Could you check a few things on this model? Use its own coordinates, in mm. A direction names the side the tool comes from. Round coordinates to 2 decimals unless told otherwise and drop trailing zeros. Loops run counter-clockwise (first coordinate to the right, second up) from the corner with the lowest first, then second, coordinate; pieces in that order, holes last. Notation, with made-up numbers: (57, 70.5) - (61, 70.5) arc R29 ccw to (61, 101.5) - close; hole circle Ø11 at (49, 80.25). An arc over 180 degrees is marked (long way). Answer as CSV lines item,"result". Start each with the question number.
1) Please list where these lines run through material, in increasing order: line 1 along X through (y, z) = (-6, 9.5); line 2 along X through (y, z) = (-16.5, 3.75); line 3 along Y through (x, z) = (7, 12.5).
2) Suppose I cut it at B-B, the plane z = 2. Write out the boundary of the cut face in (x, y).
3) Suppose I cut it at C-C, the plane x = 5. Write out the boundary of the cut face in (y, z), then the cut area to 3 significant figures.
4) We'd pull the mould along X, two halves only. Please class faces 6 (the face through (12, -16, 7)), 7 (the face through (-2, -4, 15)), 8 (the face through (-2.37, -11.7, 7.41)), 9 (the face through (-8, 0, 7)): pulls with the +X half, pulls with the -X half, needs draft (parallel to the pull), parting line crosses it, or undercut.
5) Suppose I cut it at A-A, the plane y = -4. Write out the boundary of the cut face in (x, z), then the cut area to 3 significant figures.
6) I'm going to push flat-ended pins straight in: pin 1 Ø1 at (y, z) = (9, 12.5) entering from +X; pin 2 Ø8 at (y, z) = (-17, 7) entering from -X; pin 3 Ø4 at (x, z) = (-2, 5.5) entering from -Y. Where does each tip first touch, or does it pass through?
7) Which directions (+Z, -Z, +X, -X, +Y, -Y) give clear straight access to the entire face, cutting with the end or side of a thin tool? Please do faces 1 (the face through (-4.5, -2.8, 0.5)), 2 (the face through (8.5, -16.2, 14.5)), 3 (the face through (-3.5, -10.84, 0.49)), 4 (the face through (2, -6, 7)), 5 (the face through (-1.5, -15.9, 14.5)).
```python
from build123d import *

# Parameters (mm, degrees)
F1_DEPTH = 15
F2_SIZE  = 1


with BuildPart() as f1:
    # F0 (on Top) → F1 (new body)
    with BuildSketch(Plane.XY):
        with BuildLine():
            ThreePointArc((-8, 8.423196), (-8.585786, 7.008983), (-10, 6.423196))
            Line((-10, 6.423196), (-10, -7.990119))
            Line((-10, -7.990119), (-10, -9.990119))
            ThreePointArc((-10, -9.990119), (-8.585786, -9.404332), (-8, -7.990119))
            Line((-8, -7.990119), (-8, 8.423196))
        make_face()
        with BuildLine():
            Line((-10, -7.990119), (-10, 6.423196))
            ThreePointArc((-10, 6.423196), (-11.414214, 7.008983), (-12, 8.423196))
            Line((-12, 8.423196), (-12, -7.990119))
            ThreePointArc((-12, -7.990119), (-11.414214, -9.404332), (-10, -9.990119))
            Line((-10, -9.990119), (-10, -7.990119))
        make_face()
        with BuildLine():
            Line((-10, 6.423196), (-10, 8.423196))
            ThreePointArc((-10, 8.423196), (-9.898979, 9.423196), (-9.6, 10.382788))
            ThreePointArc((-9.6, 10.382788), (-11.264911, 9.97239), (-12, 8.423196))
            ThreePointArc((-12, 8.423196), (-11.414214, 7.008983), (-10, 6.423196))
        make_face()
        with BuildLine():
            ThreePointArc((-9.6, 10.382788), (-9.898979, 9.423196), (-10, 8.423196))
            Line((-10, 8.423196), (-10, 6.423196))
            ThreePointArc((-10, 6.423196), (-8.585786, 7.008983), (-8, 8.423196))
            ThreePointArc((-8, 8.423196), (-8.450807, 9.688108), (-9.6, 10.382788))
        make_face()
        with BuildLine():
            ThreePointArc((-0.4, 10.382788), (-5, 13.423196), (-9.6, 10.382788))
            ThreePointArc((-9.6, 10.382788), (-8.450807, 9.688108), (-8, 8.423196))
            ThreePointArc((-8, 8.423196), (-5, 11.423196), (-2, 8.423196))
            ThreePointArc((-2, 8.423196), (-1.549193, 9.688108), (-0.4, 10.382788))
        make_face()
        with BuildLine():
            ThreePointArc((-12, 8.423196), (-11.264911, 9.97239), (-9.6, 10.382788))
            ThreePointArc((-9.6, 10.382788), (-5, 13.423196), (-0.4, 10.382788))
            ThreePointArc((-0.4, 10.382788), (1.264911, 9.97239), (2, 8.423196))
            ThreePointArc((2, 8.423196), (-5, 15.423196), (-12, 8.423196))
        make_face()
        with BuildLine():
            ThreePointArc((2, 8.423196), (1.264911, 9.97239), (-0.4, 10.382788))
            ThreePointArc((-0.4, 10.382788), (-0.101021, 9.423196), (0, 8.423196))
            Line((0, 8.423196), (0, 6.423196))
            ThreePointArc((0, 6.423196), (1.414214, 7.008983), (2, 8.423196))
        make_face()
        with BuildLine():
            ThreePointArc((0, 8.423196), (-0.101021, 9.423196), (-0.4, 10.382788))
            ThreePointArc((-0.4, 10.382788), (-1.549193, 9.688108), (-2, 8.423196))
            ThreePointArc((-2, 8.423196), (-1.414214, 7.008983), (0, 6.423196))
            Line((0, 6.423196), (0, 8.423196))
        make_face()
        with BuildLine():
            ThreePointArc((0, 6.423196), (-1.414214, 7.008983), (-2, 8.423196))
            ThreePointArc((-2, 8.423196), (-2.589872, 6.63678), (-4.127523, 5.552868))
            ThreePointArc((-4.127523, 5.552868), (-4.758099, 5.108366), (-5, 4.375774))
            Line((-5, 4.375774), (-5, -10.118682))
            ThreePointArc((-5, -10.118682), (-4.639662, -10.988615), (-3.769728, -11.348953))
            Line((-3.769728, -11.348953), (-3.230272, -11.348953))
            ThreePointArc((-3.230272, -11.348953), (-2.360338, -11.709292), (-2, -12.579225))
            Line((-2, -12.579225), (-2, -19.403434))
            ThreePointArc((-2, -19.403434), (-1.414214, -17.98922), (0, -17.403434))
            Line((0, -17.403434), (0, 6.423196))
        make_face()
        with BuildLine():
            Line((2, -19.403434), (2, 8.423196))
            ThreePointArc((2, 8.423196), (1.414214, 7.008983), (0, 6.423196))
            Line((0, 6.423196), (0, -17.403434))
            ThreePointArc((0, -17.403434), (1.414214, -17.98922), (2, -19.403434))
        make_face()
        with BuildLine():
            ThreePointArc((0.4, -21.363025), (1.549193, -20.668345), (2, -19.403434))
            ThreePointArc((2, -19.403434), (1.414214, -17.98922), (0, -17.403434))
            Line((0, -17.403434), (0, -19.403434))
            ThreePointArc((0, -19.403434), (0.101021, -20.403434), (0.4, -21.363025))
        make_face()
        with BuildLine():
            Line((0, -19.403434), (0, -17.403434))
            ThreePointArc((0, -17.403434), (-1.414214, -17.98922), (-2, -19.403434))
            ThreePointArc((-2, -19.403434), (-1.264911, -20.952627), (0.4, -21.363025))
            ThreePointArc((0.4, -21.363025), (0.101021, -20.403434), (0, -19.403434))
        make_face()
        with BuildLine():
            ThreePointArc((9.6, -21.363025), (5, -24.403434), (0.4, -21.363025))
            ThreePointArc((0.4, -21.363025), (-1.264911, -20.952627), (-2, -19.403434))
            ThreePointArc((-2, -19.403434), (5, -26.403434), (12, -19.403434))
            ThreePointArc((12, -19.403434), (11.264911, -20.952627), (9.6, -21.363025))
        make_face()
        with BuildLine():
            ThreePointArc((8, -19.403434), (5, -22.403434), (2, -19.403434))
            ThreePointArc((2, -19.403434), (1.549193, -20.668345), (0.4, -21.363025))
            ThreePointArc((0.4, -21.363025), (5, -24.403434), (9.6, -21.363025))
            ThreePointArc((9.6, -21.363025), (8.450807, -20.668345), (8, -19.403434))
        make_face()
        with BuildLine():
            ThreePointArc((10, -17.403434), (8.585786, -17.98922), (8, -19.403434))
            ThreePointArc((8, -19.403434), (8.450807, -20.668345), (9.6, -21.363025))
            ThreePointArc((9.6, -21.363025), (9.898979, -20.403434), (10, -19.403434))
            Line((10, -19.403434), (10, -17.403434))
        make_face()
        with BuildLine():
            ThreePointArc((10, -19.403434), (9.898979, -20.403434), (9.6, -21.363025))
            ThreePointArc((9.6, -21.363025), (11.264911, -20.952627), (12, -19.403434))
            ThreePointArc((12, -19.403434), (11.414214, -17.98922), (10, -17.403434))
            Line((10, -17.403434), (10, -19.403434))
        make_face()
        with BuildLine():
            Line((10, -13.086037), (10, -17.403434))
            ThreePointArc((10, -17.403434), (11.414214, -17.98922), (12, -19.403434))
            Line((12, -19.403434), (12, -13.086037))
            ThreePointArc((12, -13.086037), (11.414214, -11.671824), (10, -11.086037))
            Line((10, -11.086037), (10, -13.086037))
        make_face()
        with BuildLine():
            Line((8, -13.086037), (8, -19.403434))
            ThreePointArc((8, -19.403434), (8.585786, -17.98922), (10, -17.403434))
            Line((10, -17.403434), (10, -13.086037))
            Line((10, -13.086037), (10, -11.086037))
            ThreePointArc((10, -11.086037), (8.585786, -11.671824), (8, -13.086037))
        make_face()
    extrude(amount=F1_DEPTH)

    # F2
    f2_edges = [f1.edges().sort_by_distance(p)[0] for p in [
        (-5, 15.423196, 15),
        (-12, 0.216539, 15),
        (-10, -9.990119, 15),
        (-8, 0.216539, 15),
        (-3.213583, 10.833324, 15),
        (-4.758099, 5.108366, 15),
        (-5, -2.871454, 15),
        (-4.639662, -10.988615, 15),
        (-3.5, -11.348953, 15),
        (-2.360338, -11.709292, 15),
        (-2, -15.991329, 15),
        (5, -26.403434, 15),
        (12, -16.244735, 15),
        (10, -11.086037, 15),
        (8, -16.244735, 15),
        (5, -22.403434, 15),
        (2, -5.490119, 15),
        (-5, 15.423196, 0),
        (-12, 0.216539, 0),
        (-10, -9.990119, 0),
        (-8, 0.216539, 0),
        (-3.213583, 10.833324, 0),
        (-4.758099, 5.108366, 0),
        (-5, -2.871454, 0),
        (-4.639662, -10.988615, 0),
        (-3.5, -11.348953, 0),
        (-2.360338, -11.709292, 0),
        (-2, -15.991329, 0),
        (5, -26.403434, 0),
        (12, -16.244735, 0),
        (10, -11.086037, 0),
        (8, -16.244735, 0),
        (5, -22.403434, 0),
        (2, -5.490119, 0),
    ]]
    chamfer(f2_edges, length=F2_SIZE)


solid = f1.part
```
Filled sheet:
1,line 1,"-12 to -8, -5 to 2"
1,line 2,"-2 to 2, 8 to 12"
1,line 3,"-26.11 to -21.64"
2,outline,"(-12, -7.99) arc R2 ccw to (-8, -7.99) - (-8, 8.42) arc R3 cw (long way) to (-4.13, 5.55) arc R1.23 ccw to (-5, 4.38) - (-5, -10.12) arc R1.23 ccw to (-3.77, -11.35) - (-3.23, -11.35) arc R1.23 cw to (-2, -12.58) - (-2, -19.4) arc R7 ccw to (12, -19.4) - (12, -13.09) arc R2 ccw to (8, -13.09) - (8, -19.4) arc R3 cw to (2, -19.4) - (2, 8.42) arc R7 ccw to (-12, 8.42) - close"
3,outline,"(-26.4, 1) - (-25.4, 0) - (-23.4, 0) - (-22.4, 1) - (-22.4, 14) - (-23.4, 15) - (-25.4, 15) - (-26.4, 14) - close"
3,area,"58.0 mm²"
4,face 6,"pulls with the +X half"
4,face 7,"needs draft"
4,face 8,"pulls with the -X half"
4,face 9,"undercut"
5,outline,"(-12, 1) - (-11, 0) - (-9, 0) - (-8, 1) - (-8, 14) - (-9, 15) - (-11, 15) - (-12, 14) - close; (-5, 1) - (-4, 0) - (1, 0) - (2, 1) - (2, 14) - (1, 15) - (-4, 15) - (-5, 14) - close"
5,area,"161 mm²"
6,pin 1,"x = 2"
6,pin 2,"x = -2"
6,pin 3,"y = -24.3"
7,face 1,"-Z, -Y"
7,face 2,"+Z, +Y"
7,face 3,"-Z, -X, -Y"
7,face 4,"+Z, -Z, +Y"
7,face 5,"+Z, -X, -Y"
